Can you work these out from the model? Positions are in its coordinate system, mm. A direction names the side the tool comes from. Coordinates: 2 decimals unless noted, no trailing zeros. Write each loop counter-clockwise with the first axis right and the second up, starting at its lowest first coordinate (ties: lowest second). Pieces come first, ordered by that corner, then holes. Notation, with made-up numbers: (13.25, 62) -> (32.25, 62) arc R21 cw to (32.25, 72) -> close; hole circle Ø1 at (2.25, 31.5). An arc over 180 degrees is marked (long way). Use one line per item in the form item = value.
Autodesk Fusion 360 part; units mm, degrees
sketch "Sketch5" plane through (0, 0, 0) normal (0, 1, 0) x (1, 0, 0)
  line L0 (0, 0) -> (-30, 0)
  line L1 (-30, 0) -> (-30, -180)
  line L2 (-30, -180) -> (0, -180)
  line L3 (0, -180) -> (0, 0)
  dimension "d12" = 30
  dimension "d13" = 180
extrude "Extrude4" add sketch "Sketch5" along normal blind 4
sketch "Sketch6" plane through (0, 4, 0) normal (0, 1, 0) x (-1, 0, 0)
  line L0 (0, 180) -> (0, 0)
  line L1 (0, 0) -> (30, 0)
  line L2 (30, 0) -> (30, 180)
  line L3 (30, 180) -> (0, 180)
  line L4 (0, 180) -> (30, 180)
  line L5 (30, 180) -> (30, 170)
  line L6 (30, 170) -> (0, 170)
  line L7 (0, 170) -> (0, 180)
  dimension "d16" = 10
extrude "Extrude5" add sketch "Sketch6" along normal blind 106 contours L0 L2 L3 L4 L5 L6 L7
sketch "Sketch7" plane through (0, 4, 0) normal (0, 1, 0) x (-1, 0, 0)
  line L0 (30, 170) -> (0, 170)
  line L1 (0, 170) -> (0, 0)
  line L2 (0, 0) -> (30, 0)
  line L3 (30, 0) -> (30, 170)
  line L4 (0, 0) -> (30, 0)
  line L5 (30, 0) -> (30, 10)
  line L6 (30, 10) -> (0, 10)
  line L7 (0, 10) -> (0, 0)
  dimension "d19" = 10
extrude "Extrude6" add sketch "Sketch7" along normal blind 25 contours L1 L2 L3 L4 L5 L6 L7
sketch "Sketch8" plane through (-30, 0, 0) normal (-1, 0, 0) x (0, 0, 1)
  line L0 (0, 0) -> (180, 0)
  line L1 (180, 0) -> (180, 110)
  line L2 (180, 110) -> (170, 110)
  line L3 (170, 110) -> (170, 4)
  line L4 (170, 4) -> (10, 4)
  line L5 (10, 4) -> (10, 29)
  line L6 (10, 29) -> (0, 29)
  line L7 (0, 29) -> (0, 0)
  line L8 (10, 29) -> (-30, 29)
  line L9 (-30, 29) -> (-30, 35)
  line L10 (-30, 35) -> (10, 35)
  line L11 (10, 35) -> (10, 29)
  dimension "d22" = 40
  dimension "d23" = 6
extrude "Extrude7" add sketch "Sketch8" against normal blind 30 contours L6 L8 L9 L10 L11
sketch "Sketch9" plane through (-30, 0, 0) normal (-1, 0, 0) x (0, 0, 1)
  line L0 (0, 0) -> (180, 0)
  line L1 (180, 0) -> (180, 110)
  line L2 (180, 110) -> (170, 110)
  line L3 (170, 110) -> (170, 4)
  line L4 (170, 4) -> (10, 4)
  line L5 (10, 4) -> (10, 35)
  line L6 (10, 35) -> (-30, 35)
  line L7 (-30, 35) -> (-30, 29)
  line L8 (-30, 29) -> (0, 29)
  line L9 (0, 29) -> (0, 0)
  line L10 (-30, 35) -> (180, 110)
  line L11 (-30, 29) -> (180, 104)
  line L12 (180, 104) -> (180, 110)
  line L13 (-30, 35) -> (-30, 29)
extrude "Extrude8" add sketch "Sketch9" against normal blind 30 contours L3 L6 L10 L11
sketch "Sketch10" plane through (-30, 0, 0) normal (-1, 0, 0) x (0, 0, 1)
  line L0 (170, 100.4286) -> (170, 4)
  line L1 (170, 4) -> (10, 4)
  line L2 (10, 4) -> (10, 35)
  line L3 (10, 35) -> (-13.2, 35)
  line L4 (-13.2, 35) -> (170, 100.4286)
  line L5 (170, 106.4286) -> (-30, 35)
  line L6 (-30, 35) -> (-30, 29)
  line L7 (-30, 29) -> (0, 29)
  line L8 (0, 29) -> (0, 0)
  line L9 (0, 0) -> (180, 0)
  line L10 (180, 0) -> (180, 110)
  line L11 (180, 110) -> (170, 110)
  line L12 (170, 110) -> (170, 106.4286)
  line L13 (180, 110) -> (170, 106.4286)
  line L14 (170, 110) -> (180, 110)
extrude "Extrude9" cut sketch "Sketch10" against normal blind 30 contours L11 L12 L13 L14
extrude "Extrude10" add 1 faces at (-20, 4, 63.3333) along direction (0, 1, 0) blind 2
sketch "Sketch11" plane through (-30, 0, 0) normal (-1, 0, 0) x (0, 0, 1)
  line L0 (180, 110) -> (-30, 35)
  line L1 (-30, 35) -> (-30, 29)
  line L2 (-30, 29) -> (0, 29)
  line L3 (0, 29) -> (0, 0)
  line L4 (0, 0) -> (180, 0)
  line L5 (180, 0) -> (180, 110)
  line L6 (170, 6) -> (10, 6)
  line L7 (10, 6) -> (10, 35)
  line L8 (10, 35) -> (-13.2, 35)
  line L9 (-13.2, 35) -> (170, 100.4286)
  line L10 (170, 100.4286) -> (170, 6)
  line L11 (-30, 29) -> (-33, 29)
  line L12 (-33, 29) -> (-33, 48)
  line L13 (-33, 48) -> (-30, 48)
  line L14 (-30, 48) -> (-30, 29)
  dimension "d32" = 3
  dimension "d33" = 19
extrude "Extrude11" add sketch "Sketch11" against normal blind 30 contours L1 L11 L12 L13 L14
sketch "Sketch12" plane through (-30, 0, 0) normal (-1, 0, 0) x (0, 0, 1)
  line L0 (180, 110) -> (-30, 35)
  line L1 (-30, 35) -> (-30, 48)
  line L2 (-30, 48) -> (-33, 48)
  line L3 (-33, 48) -> (-33, 29)
  line L4 (-33, 29) -> (0, 29)
  line L5 (0, 29) -> (0, 0)
  line L6 (0, 0) -> (180, 0)
  line L7 (180, 0) -> (180, 110)
  line L8 (170, 6) -> (10, 6)
  line L9 (10, 6) -> (10, 35)
  line L10 (10, 35) -> (-13.2, 35)
  line L11 (-13.2, 35) -> (170, 100.4286)
  line L12 (170, 100.4286) -> (170, 6)
  line L13 (-30, 48) -> (-25.2926, 49.6855)
  line L14 (-30, 48) -> (-25, 48) construction
  line L15 (-25.2926, 49.6855) -> (-26.3039, 52.5099)
  line L16 (-26.3039, 52.5099) -> (-33, 50.1123)
  line L17 (-33, 50.1123) -> (-33, 48)
  dimension "d38" = 5
  dimension "d39" = 19.7
  dimension "d40" = 3
extrude "Extrude12" add sketch "Sketch12" against normal blind 30 contours L2 L13 L15 L16 L17
fillet "Fillet1" radius 5 1 edges at (-15, 29, -33)
fillet "Fillet2" radius 3 1 edges at (-15, 50.1123, -33)
fillet "Fillet3" radius 4 1 edges at (-15, 35, -30)
fillet "Fillet4" radius 1 2 edges at (-15, 52.5099, -26.3039) (-15, 49.6855, -25.2926)
fillet "Fillet5" radius 2 1 edges at (-15, 35, -13.2)
fillet "Fillet6" radius 5 1 edges at (-15, 110, 180)
fillet "Fillet7" radius 5 2 edges at (-15, 0, 0) (-15, 0, 180)
fillet "Fillet8" radius 5 4 edges at (-15, 35, 10) (-15, 6, 10) (-15, 100.4286, 170) (-15, 6, 170)
sketch "Sketch13" plane through (0, 6, 0) normal (0, 1, 0) x (-1, 0, 0)
  line L0 (30, 165) -> (0, 165)
  line L1 (0, 165) -> (0, 15)
  line L2 (0, 15) -> (30, 15)
  line L3 (30, 15) -> (30, 165)
  circle A0 centre (15, 50) radius 4
  circle A1 centre (15, 130) radius 4
  dimension "d59" = 8
  dimension "d61" = 8
  dimension "d62" = 80
  dimension "d63" = 35
extrude "Extrude13" cut sketch "Sketch13" against normal blind 6 contours A0 | A1
delete_face "DeleteFace1" 1 faces at (-20, 36.0576, -3.4176)
fillet "Fillet9" radius 3 1 edges at (-15, 35, -13.2)
delete_face "DeleteFace2" 1 faces at (-20, 98.2371, 165.9775)
fillet "Fillet10" radius 6 1 edges at (-15, 100.4286, 170)
Q1. Will these pins go through, and if not, where does the flat tip stop? pin 1 (1 mm diameter, centred on x = -11, z = 4.5, fed in from +Y); pin 2 (15 mm diameter, centred on x = -20, z = 82.5, fed in from +Y); pin 3 (9 mm diameter, centred on x = -15, z = 50, fed in from +Y); pin 4 (2 mm diameter, centred on x = -6.5, z = 45.5, fed in from -Y).
Return value:
pin_1 = 47.5
pin_2 = 77.86
pin_3 = 65.18
pin_4 = 0
Q2. Suppose I cut it at C-C (z = 76). Write out the boundary of the cut face in (x, y).
Return value:
outline = (-30, 0) -> (0, 0) -> (0, 6) -> (-30, 6) -> close; (-30, 66.86) -> (0, 66.86) -> (0, 72.86) -> (-30, 72.86) -> close
Q3. Thinking about a two-plate mould opening in Z: for faces 1 (the flat face through (-15, 29, -14)), 2 (the cylindrical face through (-15, 30, -31)), 3 (the flat face through (-15, 51, 170)), which applies, released by +Z, released by -Z, zero draft, split by the parting line, or undercut?
Return value:
face_1 = zero draft
face_2 = released by -Z
face_3 = undercut
Q4. Suppose I cut it at A-A (y = 73.5). Write out the boundary of the cut face in (x, z).
Return value:
outline = (-30, 77.8) -> (0, 77.8) -> (0, 94.6) -> (-30, 94.6) -> close; (-30, 170) -> (0, 170) -> (0, 180) -> (-30, 180) -> close
Q5. If I drill on line 1 (Z direction, x = -14.75, y = 16); line 2 (Z direction, x = -15, y = 1.7); line 3 (Y direction, x = -4.75, z = 63), over which ranges is the centre line in solid material (lowest first)? Write a range as from..to.
Return value:
line_1 = 0..10, 170..180
line_2 = 1.24..46, 54..126, 134..178.76
line_3 = 0..6, 62.21..68.21
Q6. For faces 4 (the flat face through (-15.21, 51.51, -29.1)), 5 (the flat face through (-15, 6, 89)), 6 (the cylindrical face through (-11.8, 3, 47.6)), which set-ups out of +Z, -Z, +X, -X, +Y, -Y let a thin tool reach every point of the face, with its end or its side?
Return value:
face_4 = -Z, +X, -X, +Y
face_5 = +X, -X
face_6 = -Y
Q7. Suppose I cut it at D-D (z = 130). Write out the boundary of the cut face in (x, y), then the cut area to 3 significant figures.
Return value:
outline = (-30, 0) -> (-19, 0) -> (-19, 6) -> (-30, 6) -> close; (-30, 86.14) -> (0, 86.14) -> (0, 92.14) -> (-30, 92.14) -> close; (-11, 0) -> (0, 0) -> (0, 6) -> (-11, 6) -> close
area = 312 mm2
